```python
from build123d import *

# Parameters (mm, degrees)
SKETCH1_R           = 7.25
SKETCH1_R_2         = 1.25
BOSS_EXTRUDE1_DEPTH = 1.75


with BuildPart() as part:
    # Sketch1 → Boss-Extrude1 (new body, symmetric)
    with BuildSketch(Plane.XY):
        Circle(SKETCH1_R)
        Circle(SKETCH1_R_2, mode=Mode.SUBTRACT)
    extrude(amount=BOSS_EXTRUDE1_DEPTH, both=True)

    # Sketch2 one side → Cut-Revolve1 (revolve, cut)
    with BuildSketch(Plane(origin=(0, 0, 0), x_dir=(1, 0, 0), z_dir=(0, 1, 0))):
        with BuildLine():
            Line((7.25, 1.75), (0, 1.75))
            Line((0, 1.75), (0, 0.619021131))
            ThreePointArc((0, 0.619021131), (3.668842229, 0.903465386), (7.25, 1.75))
        make_face()
    cut_revolve1 = revolve(axis=Axis((0, 0, -3.982137232), (0, 0, 1)), mode=Mode.SUBTRACT)

    # Mirror1: Cut-Revolve1 across plane
    add(cut_revolve1.mirror(Plane.XY), mode=Mode.SUBTRACT)


solid = part.part
```
Check sheet for the modelled part. Datum: model origin and axes. Units: mm. Round coordinates to 2 decimals unless told otherwise and drop trailing zeros. Loops run counter-clockwise (first coordinate to the right, second up) from the corner with the lowest first, then second, coordinate; pieces in that order, holes last. Notation, with made-up numbers: (59, 39.5) -> (68, 39.5) arc R16 cw to (68, 57.5) -> close; hole circle Ø8 at (-39.5, -22.5). An arc over 180 degrees is marked (long way). Write item = value, one per line. Start each with the question number.
1) Sectioned sample at B-B, the plane y = 0.5. Record the cut outline in (x, z).
2) Thickness scan on probe 1 along Y at (x, z) = (0, -0.15); probe 2 along X at (y, z) = (2.75, 0.35); probe 3 along Z at (x, y) = (2, 4.5). Record the ranges inside material, lowest first.
3) Release check for a two-part mould opening along Y. For faces 1 (the cylindrical face through (3.35, -6.43, 0.02)), 2 (the cylindrical face through (-0.27, -1.22, -0.01)) record: released by +Y, released by -Y, zero draft, split by the parting line, or undercut.
4) Gauge pin test, flat ends, axial feed: pin 1 Ø1.5 at (x, y) = (4.5, -1) entering from -Z; pin 2 Ø5 at (x, y) = (1, 0) entering from -Z; pin 3 Ø1.5 at (x, y) = (0, 0) entering from +Z. Record the tip position at first contact, or that the pin passes through.
5) Sectioned sample at C-C, the plane z = -0.1. Record the cut outline in (x, y), plus the area to 3 significant figures.
6) Sectioned sample at A-A, the plane x = 0. Record the cut outline in (y, z).
7) Sectioned sample at D-D, the plane x = 5.25. Record the cut outline in (y, z).
Results are:
q1.outline = (-7.23, -1.75) arc R23.8 cw to (-1.15, -0.65) -> (-1.15, 0.65) arc R23.8 cw to (-7.23, 1.75) -> close; (1.15, -0.65) arc R23.8 cw to (7.23, -1.75) -> (7.23, 1.75) arc R23.8 cw to (1.15, 0.65) -> close
q2.probe_1 = -7.25 to -1.25, 1.25 to 7.25
q2.probe_2 = -6.71 to 6.71
q2.probe_3 = -1.13 to 1.13
q3.face_1 = split by the parting line
q3.face_2 = undercut
q4.pin_1 = -1.23
q4.pin_2 = -0.88
q4.pin_3 = through
q5.outline = circle Ø14.5 at (0, 0); hole circle Ø2.5 at (0, 0)
q5.area = 160 mm^2
q6.outline = (-7.25, -1.75) arc R23.8 cw to (-1.25, -0.65) -> (-1.25, 0.65) arc R23.8 cw to (-7.25, 1.75) -> close; (1.25, -0.65) arc R23.8 cw to (7.25, -1.75) -> (7.25, 1.75) arc R23.8 cw to (1.25, 0.65) -> close
q7.outline = (-5, -1.75) arc R23.22 cw to (5, -1.75) -> (5, 1.75) arc R23.22 cw to (-5, 1.75) -> close
